The figure shows three views and two pictorial views of one solid part (mm, origin at its lowest corner). Answer the questions. A direction names the side the tool comes from. Give positions to 0.01 mm unless a question says otherwise; leave off trailing zeros. Order: outer loops, then holes, each group sorted by start corner. A loop starts at its lowest first (then second) coordinate and runs counter-clockwise, first axis right, second up. Notation, with made-up numbers: (12.25, 44) - (58.25, 44) arc R16 cw to (58.25, 55) - close; hole circle Ø4 at (36, 60). An arc over 180 degrees is marked (long way). Return JSON: item names as keys, results as strings. Group by question number.
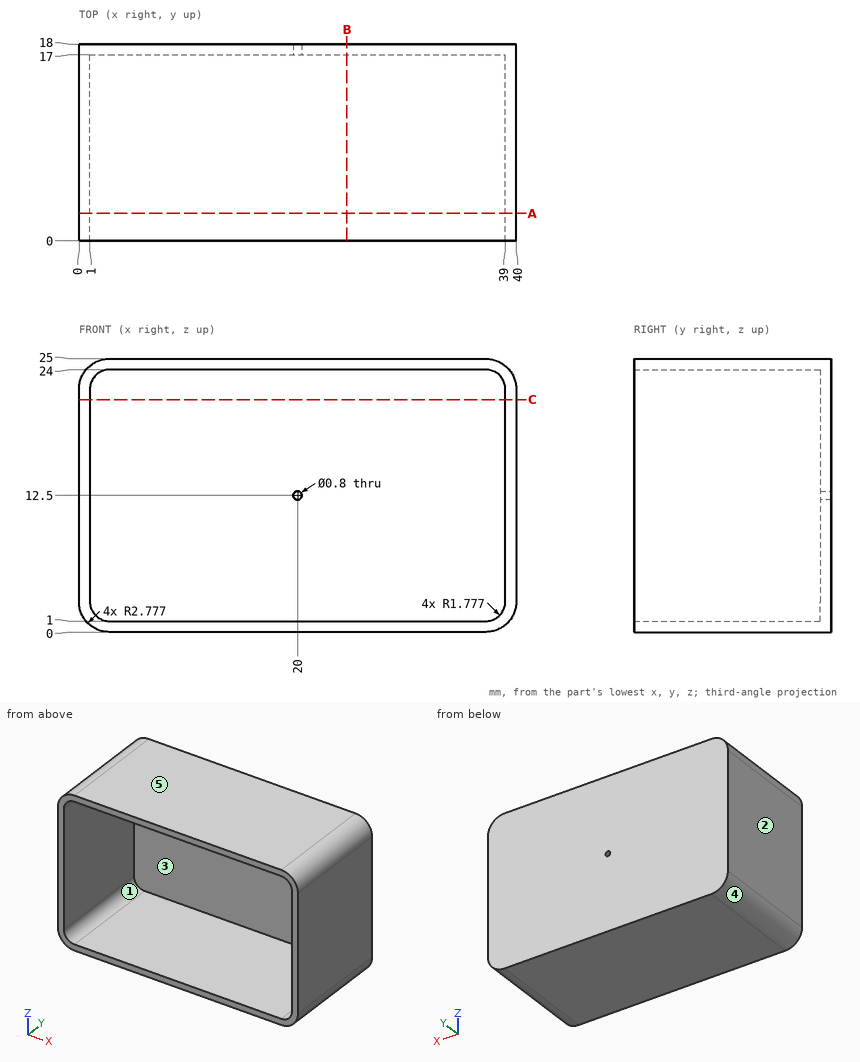
1. The part is cut by section A-A (y = 2.5). Give the vertices of the cut face in (x, z).
2. This flat-tipped pin is pushed along its axis until it touches: pin 1 (1 mm diameter, centred on y = 4, z = 3.5, fed in from -X). Where does it stop, or does it pass through?
3. A tool of negligible diameter and unlimited length cuts with its end or side. For the marked faces 1 and 2, from which of +Z, -Z, +X, -X, +Y, -Y can it reach the whole face along a straight path? Write none if from no direction.
4. The part is cut by section C-C (z = 21.25). Give the vertices of the cut face in (x, y).
5. The part is cut by section B-B (x = 24.5). Give the vertices of the cut face in (y, z), and give its area (3 significant figures).
6. Consider probe 1 along X at (y, z) = (17.4, 12.5); probe 2 along Z at (x, y) = (20, 17.4); probe 3 along X at (y, z) = (15, 21.75). Determine where each line is inside the solid, lowest interval first. Write a range as from..to.
7. Determine the mould class of the marked faces 3, 4 and 5 for opening direction X: released by +X, released by -X, zero draft, split by the parting line, or undercut.
Answers:
{
 "1": {"outline": "(0, 2.78) arc R2.78 ccw to (2.78, 0) - (37.22, 0) arc R2.78 ccw to (40, 2.78) - (40, 22.22) arc R2.78 ccw to (37.22, 25) - (2.78, 25) arc R2.78 ccw to (0, 22.22) - close; hole (1, 2.78) arc R1.78 ccw to (2.78, 1) - (37.22, 1) arc R1.78 ccw to (39, 2.78) - (39, 22.22) arc R1.78 ccw to (37.22, 24) - (2.78, 24) arc R1.78 ccw to (1, 22.22) - close"},
 "2": {"pin 1": "stops at x = 0"},
 "3": {"face 1": "-Y", "face 2": "+Z, -Z, -X, +Y, -Y"},
 "4": {"outline": "(0, 0) - (1, 0) - (1, 17) - (39, 17) - (39, 0) - (40, 0) - (40, 18) - (0, 18) - close"},
 "5": {"outline": "(0, 0) - (18, 0) - (18, 25) - (0, 25) - (0, 24) - (17, 24) - (17, 1) - (0, 1) - close", "area": "59.0 mm^2"},
 "6": {"probe 1": "x = 0..19.6, 20.4..40", "probe 2": "z = 0..12.1, 12.9..25", "probe 3": "x = 0..1, 39..40"},
 "7": {"face 3": "undercut", "face 4": "released by -X", "face 5": "zero draft"}
}
